Autodesk Inventor part; units mm, degrees
ref_plane "YZ Plane" through (0, 0, 0) normal (1, 0, 0) x (0, 1, 0)
ref_plane "XZ Plane" through (0, 0, 0) normal (0, 1, 0) x (-1, 0, 0)
ref_plane "XY Plane" through (0, 0, 0) normal (0, 0, 1) x (1, 0, 0)
sketch "Main Outline" plane through (0, 0, 0) normal (0, 0, 1) x (1, 0, 0)
  line L0 (0, 0) -> (304.8, 0) construction
  line L1 (304.8, 0) -> (304.8, 50.8) construction
  line L2 (304.8, 50.8) -> (0, 50.8) construction
  line L3 (0, 50.8) -> (0, 0) construction
  line L4 (0, 50.8) -> (0, 53.34) construction
  line L5 (0, 53.34) -> (304.8, 53.34) construction
  line L6 (304.8, 53.34) -> (304.8, 50.8) construction
  circle A0 centre (152.4, 23.8125) radius 17.4625 construction
  line L7 (152.4, 23.8125) -> (152.4, 0) construction
  circle A1 centre (152.4, 23.8125) radius 27.94 construction
  circle A2 centre (152.4, 23.8125) radius 21.59 construction
  line L8 (152.4, 23.8125) -> (144.7964, 60.3681) construction
  circle A3 centre (144.7964, 60.3681) radius 15.24 construction
  circle A4 centre (144.7964, 60.3681) radius 8.89 construction
  circle A5 centre (144.7964, 60.3681) radius 14.2875 construction
  arc A6 (164.6591, 71.8014) -> (129.0153, 43.7486) centre (144.7964, 60.3681) ccw construction
  circle A7 centre (98.8106, 85.598) radius 32.258 construction
  circle A8 centre (126.6733, 147.4971) radius 32.258 construction
  circle A9 centre (176.9075, 101.8424) radius 32.258 construction
  circle A10 centre (144.7964, 60.3681) radius 11.1125 construction
  circle A11 centre (152.4, 23.8125) radius 49.53 construction
  line L9 (144.7964, 60.3681) -> (126.6733, 147.4971) construction
  line L10 (144.7964, 60.3681) -> (98.8106, 85.598) construction
  line L11 (98.8106, 85.598) -> (176.9075, 101.8424) construction
  line L12 (176.9075, 101.8424) -> (144.7964, 60.3681) construction
  circle A12 centre (98.8106, 85.598) radius 9.5493 construction
  arc A13 (174.9629, 111.1915) -> (185.6989, 98.1139) centre (176.9075, 101.8424) ccw construction
  circle A14 centre (126.6733, 147.4971) radius 9.5493 construction
  line L13 (96.8659, 94.9472) -> (174.9629, 111.1915) construction
  line L14 (185.6989, 98.1139) -> (165.8956, 51.4198) construction
  line L15 (92.2351, 78.6732) -> (129.0153, 43.7486) construction
  line L16 (174.9629, 111.1915) -> (176.9075, 101.8424) construction
  line L17 (176.9075, 101.8424) -> (185.6989, 98.1139) construction
  arc A15 (185.6989, 98.1139) -> (174.9629, 111.1915) centre (176.9075, 101.8424) ccw construction
  arc A16 (165.8956, 51.4198) -> (164.6591, 71.8014) centre (144.7964, 60.3681) ccw construction
  arc A17 (129.0153, 43.7486) -> (165.8956, 51.4198) centre (144.7964, 60.3681) ccw construction
  circle A18 centre (126.6086, 147.808) radius 32.258 construction
  circle A19 centre (126.544, 148.1188) radius 32.258 construction
  circle A20 centre (126.4793, 148.4297) radius 32.258 construction
  line L18 (126.6733, 147.4971) -> (126.4793, 148.4297) construction
  circle A21 centre (126.738, 147.1863) radius 32.258 construction
  circle A22 centre (117.4622, 43.2997) radius 9.525 construction
  circle A23 centre (176.6694, 55.615) radius 9.525 construction
  line L19 (152.4, 23.8125) -> (117.4622, 43.2997) construction
  line L20 (152.4, 23.8125) -> (176.6694, 55.615) construction
  line L21 (117.4622, 43.2997) -> (98.8106, 85.598) construction
  line L22 (176.6694, 55.615) -> (176.9075, 101.8424) construction
  circle A24 centre (135.1821, 106.5897) radius 7.9375 construction
  line L23 (135.6243, 150.8242) -> (166.2787, 68.353) construction
  circle A25 centre (152.4, 23.8125) radius 29.845 construction
  line L24 (117.1381, 146.979) -> (121.9118, 59.1246) construction
  circle A26 centre (99.0889, 85.4453) radius 32.258 construction
  circle A27 centre (97.9755, 86.0562) radius 32.258 construction
  line L25 (97.9755, 86.0562) -> (98.8106, 85.598) construction
  circle A28 centre (98.2538, 85.9034) radius 32.258 construction
  circle A29 centre (98.5322, 85.7507) radius 32.258 construction
  circle A30 centre (152.4, 23.8125) radius 29.845 construction
  circle A31 centre (122.555, 23.8125) radius 6.35 construction
  circle A32 centre (179.7696, 35.7133) radius 6.35 construction
  line L26 (122.555, 23.8125) -> (152.4, 23.8125) construction
  line L27 (152.4, 23.8125) -> (182.245, 23.8125) construction
  circle A33 centre (182.245, 23.8125) radius 6.35 construction
  circle A34 centre (125.0304, 11.9117) radius 6.35 construction
  circle A35 centre (150.4199, 33.3321) radius 39.5684 construction
  line L28 (72.9795, 65.6655) -> (119.7593, 8.3204) construction
  circle A36 centre (177.4906, 102.5955) radius 32.258 construction
  line L29 (176.9075, 101.8424) -> (177.4906, 102.5955) construction
  circle A37 centre (177.2963, 102.3445) radius 32.258 construction
  circle A38 centre (177.1019, 102.0934) radius 32.258 construction
  circle A39 centre (176.7131, 101.5913) radius 32.258 construction
  line L30 (188.5109, 22.6209) -> (208.5442, 93.8632) construction
  circle A40 centre (135.1821, 106.5897) radius 9.5727 construction
  arc A41 (86.8202, 116.3239) -> (96.3065, 136.4856) centre (81.3304, 131.2195) ccw construction
  arc A42 (158.9123, 149.5077) -> (175.6513, 134.801) centre (174.7462, 150.6502) ccw construction
  line L31 (126.4793, 148.4297) -> (126.9966, 145.9429) construction
  line L32 (116.5322, 146.3607) -> (117.0495, 143.8739) construction
  line L33 (136.9437, 148.0119) -> (136.4264, 150.4987) construction
  arc A43 (136.4264, 150.4987) -> (116.5322, 146.3607) centre (126.4793, 148.4297) ccw construction
  arc A44 (117.0495, 143.8739) -> (136.9437, 148.0119) centre (126.9966, 145.9429) ccw construction
  line L34 (177.4906, 102.5955) -> (175.9357, 100.5871) construction
  line L35 (169.4571, 108.8154) -> (167.9021, 106.807) construction
  line L36 (183.9692, 94.3672) -> (185.5242, 96.3756) construction
  arc A45 (185.5242, 96.3756) -> (169.4571, 108.8154) centre (177.4906, 102.5955) ccw construction
  arc A46 (167.9021, 106.807) -> (183.9692, 94.3672) centre (175.9357, 100.5871) ccw construction
  line L37 (97.9755, 86.0562) -> (100.2023, 84.8344) construction
  line L38 (93.0884, 77.1487) -> (95.3153, 75.927) construction
  line L39 (105.0894, 93.7418) -> (102.8625, 94.9636) construction
  arc A47 (102.8625, 94.9636) -> (93.0884, 77.1487) centre (97.9755, 86.0562) ccw construction
  arc A48 (95.3153, 75.927) -> (105.0894, 93.7418) centre (100.2023, 84.8344) ccw construction
  circle A49 centre (117.4622, 43.2997) radius 3.9687 construction
  circle A50 centre (176.6694, 55.615) radius 3.9687 construction
  line L40 (152.4, 23.8125) -> (158.4777, -5.4071) construction
  arc A51 (89.4797, 54.6517) -> (86.0737, 49.6139) centre (88.534, 51.6209) ccw construction
  arc A52 (202.9367, 73.9217) -> (197.8043, 77.1835) centre (199.8802, 74.7812) ccw construction
  circle A53 centre (152.4, 23.8125) radius 14.224 construction
  circle A54 centre (135.1821, 106.5897) radius 3.9687 construction
  circle A55 centre (156.538, 3.9183) radius 6.35 construction
  circle A56 centre (156.538, 3.9183) radius 2.0828 construction
  circle A57 centre (152.4, 23.8125) radius 20.32 construction
  line L41 (133.1021, 30.1759) -> (152.4, 23.8125) construction
  line L42 (152.4, 23.8125) -> (167.5599, 37.3432) construction
  circle A58 centre (167.5599, 37.3432) radius 2.0828 construction
  circle A59 centre (167.5599, 37.3432) radius 3.9687 construction
  circle A60 centre (133.1021, 30.1759) radius 2.0828 construction
  circle A61 centre (133.1021, 30.1759) radius 3.9688 construction
  point P0 (126.738, 147.1863)
  point P1 (176.7131, 101.5913)
  dimension "d18" = 99.06
  dimension "d58" = 64.516
  dimension "d86" = 64.516
  dimension "d0" = 304.8
  dimension "d1" = 50.8
  dimension "d2" = 2.54
  dimension "d3" = 34.925
  dimension "d4" = 23.8125
  dimension "d5" = 152.4
  dimension "d6" = 55.88
  dimension "d7" = 43.18
  dimension "d8" = 37.338
  dimension "d10" = 30.48
  dimension "d11" = 17.78
  dimension "d12" = 28.575
  dimension "d13" = 45.8366
  dimension "d14" = 64.516
  dimension "d15" = 64.516
  dimension "d16" = 64.516
  dimension "d17" = 22.225
  dimension "d19" = 52.4523
  dimension "d20" = 88.9939
  dimension "d21" = 19.0986
  dimension "d22" = 19.0986
  dimension "d23" = 19.0986
  dimension "d30" = 124.732
  dimension "d40" = 64.516
  dimension "d41" = 64.516
  dimension "d42" = 64.516
  dimension "d43" = 0.9525
  dimension "d44" = 0.3175
  dimension "d45" = 0.635
  dimension "d46" = 64.516
  dimension "d47" = 0.3175
  dimension "d48" = 19.05
  dimension "d49" = 19.05
  dimension "d50" = 40.005
  dimension "d51" = 40.005
  dimension "d52" = 46.228
  dimension "d54" = 46.228
  dimension "d55" = 15.875
  dimension "d56" = 41.4655
  dimension "d57" = 59.69
  dimension "d59" = 64.516
  dimension "d60" = 64.516
  dimension "d61" = 64.516
  dimension "d62" = 0.3175
  dimension "d63" = 0.3175
  dimension "d64" = 0.635
  dimension "d65" = 0.9525
  dimension "d73" = 12.7
  dimension "d74" = 12.7
  dimension "d76" = 59.69
  dimension "d78" = 12.7
  dimension "d79" = 12.7
  dimension "d80" = 64.516
  dimension "d81" = 0.9525
  dimension "d82" = 64.516
  dimension "d83" = 64.516
  dimension "d84" = 0.3175
  dimension "d85" = 0.635
  dimension "d88" = 0.3175
  dimension "d89" = 31.75
  dimension "d90" = 31.75
  dimension "d94" = 1.5875
  dimension "d95" = 20.32
  dimension "d96" = 1.5875
sketch "Upper CIM C-C Check" plane through (0, 0, 0) normal (0, 0, 1) x (1, 0, 0)
  arc A0 (3.4429, -22.6582) -> (3.4429, 22.6582) centre (0, 0) ccw construction
  arc A1 (90.4285, 9.4409) -> (90.4285, -9.4409) centre (88.9939, 0) ccw construction
  line L0 (88.9939, 0) -> (0, 0) construction
  line L1 (90.4285, 9.4409) -> (3.4429, 22.6582)
  line L2 (3.4429, -22.6582) -> (90.4285, -9.4409)
  arc A2 (90.4285, -9.4409) -> (90.4285, 9.4409) centre (88.9939, 0) ccw
  arc A3 (3.4429, 22.6582) -> (3.4429, -22.6582) centre (0, 0) ccw
  dimension "d24" = 45.8366
  dimension "d25" = 19.0986
  dimension "d26" = 78.9119
  dimension "d27" = 87.984
  dimension "d28" = 27.12
  dimension "d29" = 88.9939
sketch "Sketch3" plane through (0, 0, 0) normal (0, 0, 1) x (1, 0, 0)
  line L0 (96.8659, 94.9472) -> (174.9629, 111.1915)
  line L1 (185.6989, 98.1139) -> (165.8956, 51.4198)
  line L2 (92.2351, 78.6732) -> (129.0153, 43.7486)
  arc A0 (96.8659, 94.9472) -> (92.2351, 78.6732) centre (98.8106, 85.598) ccw
  arc A1 (185.6989, 98.1139) -> (174.9629, 111.1915) centre (176.9075, 101.8424) ccw
  arc A2 (129.0153, 43.7486) -> (165.8956, 51.4198) centre (144.7964, 60.3681) ccw
  line L3 (175.1698, 110.1968) -> (97.0728, 93.9525)
  arc A3 (97.0728, 93.9525) -> (92.9347, 79.41) centre (98.8106, 85.598) ccw
  line L4 (92.9347, 79.41) -> (129.7149, 44.4854)
  arc A4 (129.7149, 44.4854) -> (164.9602, 51.8165) centre (144.7964, 60.3681) ccw
  line L5 (164.9602, 51.8165) -> (184.7635, 98.5106)
  arc A5 (184.7635, 98.5106) -> (175.1698, 110.1968) centre (176.9075, 101.8424) ccw
  line L6 (174.7042, 112.4349) -> (96.6073, 96.1906)
  arc A6 (96.6073, 96.1906) -> (91.3606, 77.7523) centre (98.8106, 85.598) ccw
  line L7 (91.3606, 77.7523) -> (128.1408, 42.8276)
  arc A7 (128.1408, 42.8276) -> (167.0648, 50.9239) centre (144.7964, 60.3681) ccw
  line L8 (167.0648, 50.9239) -> (186.8681, 97.618)
  arc A8 (186.8681, 97.618) -> (174.7042, 112.4349) centre (176.9075, 101.8424) ccw
  point P0 (0, 0)
  dimension "d115" = 1.27
  dimension "d116" = 1.016
extrude "Extrusion1" add sketch "Sketch3" along normal blind 4.5 contours A8 L8 A7 L7 A6 L6
extrude "Extrusion2" add sketch "Sketch3" along normal blind 4.45 contours L0 A1 L1 A2 L2 A0
mirror "Mirror1" about plane through (140.8105, 79.5306, 0) normal (0, 0, -1)
equation "\"d3\" = r10"
equation "\"d6\" = g44"
equation "\"d7\" = g34"
equation "\"d10\" = g24"
equation "\"d11\" = g14"
equation "\"d12\" = r8"
equation "\"d13\" = p48"
equation "\"d14\" = cim"
equation "\"d15\" = cim"
equation "\"d16\" = cim"
equation "\"d17\" = r6"
equation "\"d21\" = p20"
equation "\"d22\" = p20"
equation "\"d23\" = p20"
equation "\"d24\" = p48"
equation "\"d25\" = p20"
equation "\"d29\" = d20"
equation "\"g14\" = 17.78"
equation "\"g24\" = 30.48"
equation "\"g34\" = 43.18"
equation "\"g44\" = 55.88"
equation "\"p20\" = 19.09859"
equation "\"p48\" = 45.83662"
equation "\"r10\" = 34.925"
equation "\"r9\" = 31.75"
equation "\"r8\" = 28.575"
equation "\"r7\" = 25.4"
equation "\"r6\" = 22.225"
equation "\"r5\" = 19.05"
equation "\"r4\" = 15.875"
equation "\"r3\" = 12.7"
equation "\"cim\" = 64.516"
equation "\"act\" = 28.448"
equation "\"actL\" = 23.749"
equation "\"UpperCimCCCheck\" = 2 * d27 + d26 + d28"
equation "\"LowerBeltPathCCCheck\" = 267"
properties material "Rubber"
Geometry check sheet. Reference: the model listing, model coordinates, mm. A direction names the side the tool comes from. Round coordinates to 2 decimals unless told otherwise and drop trailing zeros. Order: outer loops, then holes, each group sorted by start corner. A loop starts at its lowest first (then second) coordinate and runs counter-clockwise, first axis right, second up. Notation, with made-up numbers: (-27.5, 2.25) - (-16.5, 2.25) arc R12 ccw to (-16.5, 6.25) - close; hole circle Ø6 at (17, -2). An arc over 180 degrees is marked (long way). Use a Markdown table: item, result. Add a question column.
(1) Tool access check on faces 1 (the flat face through (134, 103, -4.5)), 2 (the flat face through (174.723, 74.837, -0.062)). Record the directions out of +Z, -Z, +X, -X, +Y, -Y that give a thin tool (end or side, any length) a straight path to the whole face; none if there is none.
(2) Sectioned sample at B-B, the plane y = 83.5. Enter the section's corners in (x, z).
(3) Material ranges on line 1 along Y through (x, z) = (180, 1.75); line 2 along Y through (x, z) = (98, 1.25); line 3 along X through (y, z) = (58.5, -3), recorded low to high. Write a range as [from, to].
(4) Release check for a two-part mould opening along Y. For faces 3 (the flat face through (136.202, 104.426, -0.063)), 4 (the flat face through (109.493, 60.534, -0.063)), 5 (the flat face through (136.67, 102.19, -0.06)) record: pulls with the +Y half, pulls with the -Y half, needs draft (parallel to the pull), parting line crosses it, or undercut.
(5) Sectioned sample at A-A, the plane x = 171.5. Enter the section's corners in (y, z).
(6) Depth check by flat-ended pin: pin 1 (22 mm diameter, centred on x = 140.5, y = 86.5, fed in from -Z); pin 2 (3 mm diameter, centred on y = 78.5, z = 1, fed in from +X); pin 3 (4 mm diameter, centred on y = 57, z = -2, fed in from +X). Enter the tip coordinate at first touch or a pass-through.
(7) Sectioned sample at C-C, the plane z = 0. Enter the section's corners in (x, y), and give its area (3 significant figures).
Answers below:
| question | item | result |
|---|---|---|
| 1 | face 1 | -Z, +X, -X, +Y, -Y |
| 1 | face 2 | +Z, -Z |
| 2 | outline | (88.2, -4.5) - (89.49, -4.5) - (89.49, -4.45) - (90.54, -4.45) - (90.54, 4.45) - (89.49, 4.45) - (89.49, 4.5) - (88.2, 4.5) - close; (178.4, -4.45) - (179.5, -4.45) - (179.5, -4.5) - (180.88, -4.5) - (180.88, 4.5) - (179.5, 4.5) - (179.5, 4.45) - (178.4, 4.45) - close |
| 3 | line 1 | [81.42, 87.28], [109.8, 112.21] |
| 3 | line 2 | [71.45, 74.6], [94.15, 96.48] |
| 3 | line 3 | [111.64, 114.96], [167.79, 170.28] |
| 4 | face 3 | pulls with the +Y half |
| 4 | face 4 | pulls with the -Y half |
| 4 | face 5 | undercut |
| 5 | outline | (61.38, -4.5) - (64.63, -4.5) - (64.63, -4.45) - (67.24, -4.45) - (67.24, 4.45) - (64.63, 4.45) - (64.63, 4.5) - (61.38, 4.5) - close; (109.43, -4.45) - (110.47, -4.45) - (110.47, -4.5) - (111.77, -4.5) - (111.77, 4.5) - (110.47, 4.5) - (110.47, 4.45) - (109.43, 4.45) - close |
| 6 | pin 1 | through |
| 6 | pin 2 | x = 179.4 |
| 6 | pin 3 | x = 170.49 |
| 7 | outline | (91.36, 77.75) - (128.14, 42.83) arc R24.19 ccw to (167.06, 50.92) - (186.87, 97.62) arc R10.82 ccw to (174.7, 112.43) - (96.61, 96.19) arc R10.82 ccw to start; hole (92.93, 79.41) - (129.71, 44.49) arc R21.9 ccw to (164.96, 51.82) - (184.76, 98.51) arc R8.53 ccw to (175.17, 110.2) - (97.07, 93.95) arc R8.53 ccw to start |
| 7 | area | 612 mm² |
